Read the model definition and answer for the solid it produces. Units are mm, in the model's axes. A direction names the side the tool comes from. Coordinates: 2 decimals unless noted, no trailing zeros. Write each loop counter-clockwise with the first axis right and the second up, starting at its lowest first coordinate (ties: lowest second). Pieces come first, ordered by that corner, then holes. Notation, with made-up numbers: (60.5, -14.75) -> (119.5, -14.75) arc R22 ccw to (119.5, 7.25) -> close; hole circle Ø6 at (72, 20). An arc over 180 degrees is marked (long way). Use CSV: the item, a comma, the result in double quotes.
from build123d import *

# Parameters (mm, degrees)
BOSS_EXTRUDE1_DEPTH = 5
SKETCH2_W           = 2
SKETCH2_H           = 7.001972448
BOSS_EXTRUDE2_DEPTH = 4.5
FILLET1_R           = 4


with BuildPart() as part:
    # Sketch1 → Boss-Extrude1 (new body)
    with BuildSketch(Plane.XY):
        Polygon((0, 0), (0, 15), (2, 15), (2, 4.971605765), (2, -17), (0, -17), align=None)
    extrude(amount=BOSS_EXTRUDE1_DEPTH)

    # Sketch2 → Boss-Extrude2 (add)
    with BuildSketch(Plane(origin=(0, 0, 0), x_dir=(-1, 0, 0), z_dir=(0, 0, -1))):
        with Locations((-1, -13.499013776)):
            Rectangle(SKETCH2_W, SKETCH2_H)
    extrude(amount=BOSS_EXTRUDE2_DEPTH)

    # Fillet1
    fillet1_edges = [part.edges().sort_by_distance(p)[0] for p in [
        (1, -9.998027552, 0),
        (1, -17, 5),
    ]]
    fillet(fillet1_edges, radius=FILLET1_R)


solid = part.part
1. A tool of negligible diameter and unlimited length cuts with its end or side. For faces 1 (the flat face through (1, 5, 0)), 2 (the flat face through (2, -1, 1)), from which of +Z, -Z, +X, -X, +Y, -Y can it reach the whole face along a straight path? Write none if from no direction.
Solutions:
face 1,"-Z, +X, -X, +Y"
face 2,"+Z, -Z, +X, +Y, -Y"
2. A cutting plane is placed at C-C (z = 4). Give the vertices of the cut face in (x, y).
Solutions:
outline,"(0, -15.65) -> (2, -15.65) -> (2, 15) -> (0, 15) -> close"
3. A cutting plane is placed at B-B (y = -5). Give the vertices of the cut face in (x, z).
Solutions:
outline,"(0, 0) -> (2, 0) -> (2, 5) -> (0, 5) -> close"
4. Each of these flat-tipped pins is pushed along its axis until it touches: pin 1 Ø1 at (x, z) = (1, -2) entering from +Y; pin 2 Ø5 at (y, z) = (10.5, -1.5) entering from -X. Where does it stop, or does it pass through?
Solutions:
pin 1,"stops at y = -9.12"
pin 2,"stops at x = 0"
5. Find the intervals of material crossed by line 1 along Z through (x, y) = (0.3, 11.5); line 2 along Z through (x, y) = (1.45, -7.5); line 3 along Y through (x, z) = (0.1, 2.5), in increasing order.
Solutions:
line 1,"z = 0 to 5"
line 2,"z = -0.29 to 5"
line 3,"y = -16.71 to 15"
6. A cutting plane is placed at A-A (x = 1.5). Give the vertices of the cut face in (y, z).
Solutions:
outline,"(-17, -4.5) -> (-10, -4.5) -> (-10, -4) arc R4 cw to (-6, 0) -> (15, 0) -> (15, 5) -> (-13, 5) arc R4 ccw to (-17, 1) -> close"
